Check sheet for the modelled part. Datum: model origin and axes. Units: mm. A direction names the side the tool comes from. Round coordinates to 2 decimals unless told otherwise and drop trailing zeros. Order: outer loops, then holes, each group sorted by start corner. A loop starts at its lowest first (then second) coordinate and runs counter-clockwise, first axis right, second up. Notation, with made-up numbers: (80.5, 71) -> (89.5, 71) arc R20 cw to (89.5, 82) -> close; hole circle Ø3 at (43, -34.75). An arc over 180 degrees is marked (long way). Answer in a Markdown table with one row per item.
from build123d import *

# Parameters (mm, degrees)
PAD_DEPTH       = 12
POCKET_DEPTH    = 62
SKETCH019_W     = 31
SKETCH019_H     = 21.780884
POCKET002_DEPTH = 17
SKETCH020_R     = 2
POCKET003_DEPTH = 4
CYLINDER_R      = 4
CYLINDER_DEPTH  = 28
POCKET032_DEPTH = 5


with BuildPart() as part:
    # Sketch010 → Pad (new body, symmetric)
    with BuildSketch(Plane.XY):
        with BuildLine():
            Line((12.639868, 59.984547), (-12.639868, 59.984547))
            Line((-12.639868, 59.984547), (-17.867889, 82.058411))
            Line((-17.867889, 82.058411), (-17.867889, 102.222236))
            ThreePointArc((-15.867889, 104.222236), (-17.282103, 103.63645), (-17.867889, 102.222236))
            Line((-15.867889, 104.222236), (-8.154342, 104.222236))
            ThreePointArc((-7.154342, 103.222236), (-7.447235, 103.929343), (-8.154342, 104.222236))
            Line((-7.154342, 103.222236), (-7.154342, 92.189331))
            Line((-7.154342, 92.189331), (7.154342, 92.189331))
            Line((7.154342, 92.189331), (7.154342, 103.222236))
            ThreePointArc((8.154342, 104.222236), (7.447235, 103.929343), (7.154342, 103.222236))
            Line((8.154342, 104.222236), (15.867889, 104.222236))
            ThreePointArc((17.867889, 102.222236), (17.282103, 103.63645), (15.867889, 104.222236))
            Line((17.867889, 102.222236), (17.867889, 82.058411))
            Line((17.867889, 82.058411), (12.639868, 59.984547))
        make_face()
    extrude(amount=PAD_DEPTH, both=True)

    # Sketch011 → Pocket (cut)
    with BuildSketch(Plane.XZ.offset(-54)):
        Polygon((0, 13.813917), (-22.117895, 13.813917), (-22.117895, -0.189388), (-22.117895, -17.743416), (0, -17.743416), (22.658901, -17.743416), (22.658901, -0.111897), (22.658901, 13.813917), align=None)
        Polygon((-18.596464, 0), (-18.596464, 5.287208), (-8.154342, 8), (-7.443202, 8.179805), (0, 8.179805), (7.519913, 8.179805), (8.154342, 8), (18.531284, 5.287208), (18.531284, -0.112287), (18.531284, -5.399495), (8.154342, -8), (7.554242, -8.253323), (0.11104, -8.253323), (-7.443202, -8.253323), (-8.154342, -8), (-18.596464, -5.371119), align=None, mode=Mode.SUBTRACT)
    extrude(amount=-POCKET_DEPTH, mode=Mode.SUBTRACT)

    # Sketch019 → Pocket002 (cut)
    with BuildSketch(Plane.XY.offset(0.8)):
        with Locations((0.01352, 95.005211)):
            Rectangle(SKETCH019_W, SKETCH019_H)
    extrude(amount=-POCKET002_DEPTH, mode=Mode.SUBTRACT)

    # Sketch020 → Pocket003 (cut)
    with BuildSketch(Plane.XY.offset(0.8)):
        with Locations((-11.1, 94.9)):
            Circle(SKETCH020_R)
        with Locations((11.3, 94.9)):
            Circle(SKETCH020_R)
        with Locations((0.013518, 88.3)):
            Circle(SKETCH020_R)
    extrude(amount=POCKET003_DEPTH, mode=Mode.SUBTRACT)

    # Cylinder → Cylinder (cut)
    with BuildSketch(Plane.XZ.offset(-85)):
        Circle(CYLINDER_R)
    extrude(amount=CYLINDER_DEPTH, mode=Mode.SUBTRACT)

    # Sketch067 → Pocket032 (cut)
    with BuildSketch(Plane.XY.offset(7)):
        Polygon((-7.9, 79.180206), (0, 64.83), (7.9, 79.180206), (0, 93.53), align=None)
    extrude(amount=POCKET032_DEPTH, mode=Mode.SUBTRACT)


solid = part.part
Item 1: Cross-section at D-D (x = 12). Record the boundary of the cut face in (y, z).
Result sheet:
| item | result |
|---|---|
| outline | (59.98, -7.04) -> (84.11, -7.04) -> (84.11, 0.8) -> (93.03, 0.8) -> (93.03, 4.8) -> (96.77, 4.8) -> (96.77, 0.8) -> (104.22, 0.8) -> (104.22, 6.99) -> (59.98, 6.99) -> close |
Item 2: Set-up check for faces 1 (the flat face through (15.514, 94, -3)), 2 (the cylindrical face through (-0.867, 72.667, -3.905)), 3 (the flat face through (-7.154, 98, 5)): record each of +Z, -Z, +X, -X, +Y, -Y from which the full face is reachable in a straight line by a thin tool's end or side.
Result sheet:
| item | result |
|---|---|
| face 1 | -Z, +Y |
| face 2 | -Y |
| face 3 | +Z, -Z, +Y |
Item 3: Cross-section at A-A (y = 94.9). Record the boundary of the cut face in (x, z), and give its area (3 significant figures).
Result sheet:
| item | result |
|---|---|
| outline | (-17.87, -5.55) -> (-15.49, -6.15) -> (-15.49, 0.8) -> (-13.1, 0.8) -> (-13.1, 4.8) -> (-9.1, 4.8) -> (-9.1, 0.8) -> (-7.15, 0.8) -> (-7.15, 8.18) -> (-7.44, 8.18) -> (-8.15, 8) -> (-17.87, 5.48) -> close; (7.15, 0.8) -> (9.3, 0.8) -> (9.3, 4.8) -> (13.3, 4.8) -> (13.3, 0.8) -> (15.51, 0.8) -> (15.51, -6.16) -> (17.87, -5.57) -> (17.87, 5.46) -> (8.15, 8) -> (7.52, 8.18) -> (7.15, 8.18) -> close |
| area | 129 mm^2 |
Item 4: Mould release check, pull along Y, two halves, no side actions. Record for faces 4 (the flat face through (-17.868, 92, 0)), 5 (the flat face through (0, 88, 4.8)), 6 (the cylindrical face through (17.3, 103.62, 0.04)): pulls with the +Y half, pulls with the -Y half, needs draft (parallel to the pull), parting line crosses it, or undercut.
Result sheet:
| item | result |
|---|---|
| face 4 | needs draft |
| face 5 | undercut |
| face 6 | pulls with the +Y half |
Item 5: Scan lines: line 1 (Y direction, x = -11.1, z = 2.8); line 2 (X direction, y = 100.5, z = 0); line 3 (Y direction, x = 7, z = -0.5). Record each from-to range of solid material in increasing order. Write a range as [from, to].
Result sheet:
| item | result |
|---|---|
| line 1 | y = [59.98, 92.9], [96.9, 104.22] |
| line 2 | x = [-17.87, -15.49], [15.51, 17.87] |
| line 3 | y = [59.98, 84.11] |
Item 6: Cross-section at B-B (z = 0). Record the boundary of the cut face in (x, y).
Result sheet:
| item | result |
|---|---|
| outline | (-17.87, 82.06) -> (-12.64, 59.98) -> (-4, 59.98) -> (-4, 84.11) -> (-15.49, 84.11) -> (-15.49, 104.22) -> (-15.87, 104.22) arc R2 ccw to (-17.87, 102.22) -> close; (4, 59.98) -> (12.64, 59.98) -> (17.87, 82.06) -> (17.87, 102.22) arc R2 ccw to (15.87, 104.22) -> (15.51, 104.22) -> (15.51, 84.11) -> (4, 84.11) -> close |
Item 7: Cross-section at C-C (z = 3.5). Record the boundary of the cut face in (x, y), and give its area (3 significant figures).
Result sheet:
| item | result |
|---|---|
| outline | (-17.87, 82.06) -> (-12.64, 59.98) -> (-1.94, 59.98) -> (-1.94, 85) -> (1.94, 85) -> (1.94, 59.98) -> (12.64, 59.98) -> (17.87, 82.06) -> (17.87, 102.22) arc R2 ccw to (15.87, 104.22) -> (8.15, 104.22) arc R1 ccw to (7.15, 103.22) -> (7.15, 92.19) -> (-7.15, 92.19) -> (-7.15, 103.22) arc R1 ccw to (-8.15, 104.22) -> (-15.87, 104.22) arc R2 ccw to (-17.87, 102.22) -> close; hole circle Ø4 at (-11.1, 94.9); hole circle Ø4 at (0.01, 88.3); hole circle Ø4 at (11.3, 94.9) |
| area | 1,160 mm^2 |
Item 8: Depth check by flat-ended pin: P1, Ø2, axis at x = 4, z = 1, coming from the +Y side; P2, Ø1.6, axis at x = -1, z = 2.5, coming from the -Y side; P3, Ø2, axis at x = 0.5, y = 88, coming from the -Z side; P4, Ø4, axis at x = -2.5, y = 94.5, coming from the +Z side. Enter the tip coordinate at first touch or a pass-through.
Result sheet:
| item | result |
|---|---|
| P1 | stops at y = 92.19 |
| P2 | stops at y = 85 |
| P3 | stops at z = 4.8 |
| P4 | passes through |
